Design review of the part shown in the three views and the two pictorial views. Dimensions are in mm from the part's minimum x, y and z. Round coordinates to 2 decimals unless told otherwise and drop trailing zeros. Order: outer loops, then holes, each group sorted by start corner. A loop starts at its lowest first (then second) coordinate and runs counter-clockwise, first axis right, second up.
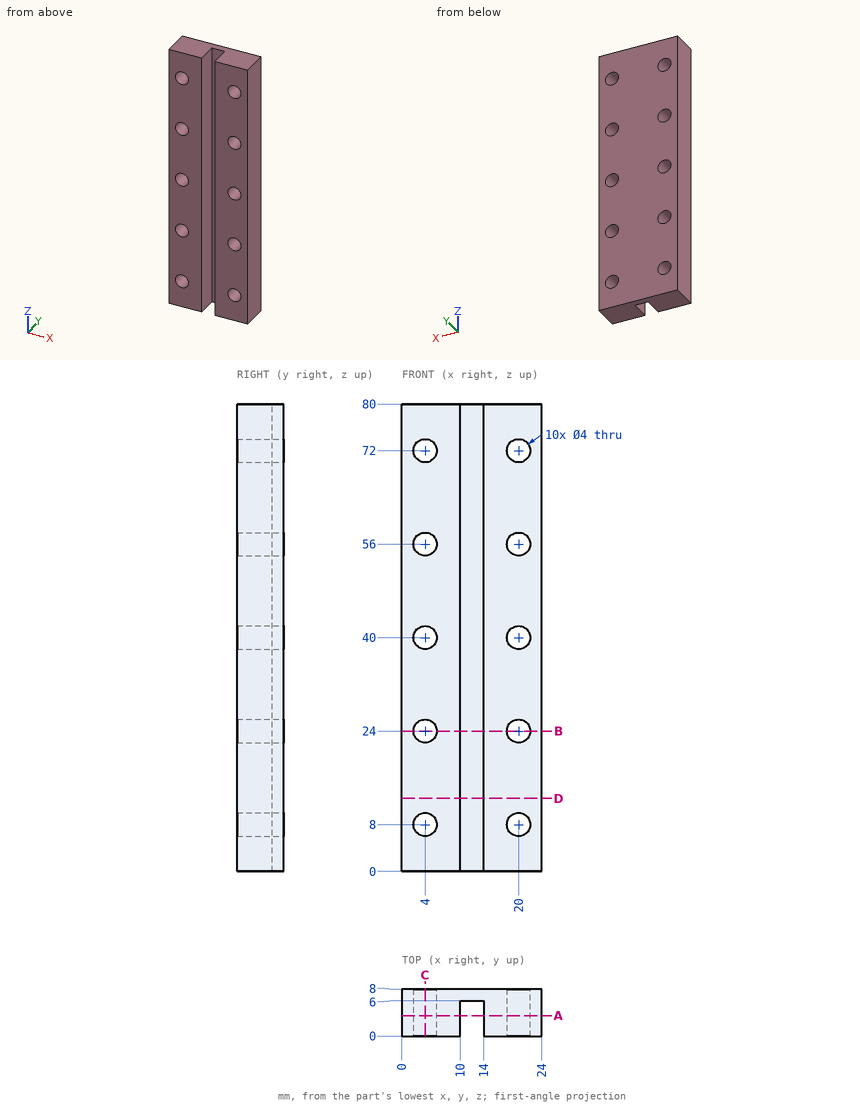
(1) Clearance check with flat-ended pins moving along their axes: P1, Ø3.5, axis at x = 4, z = 40, coming from the +Y side; P2, Ø1.2, axis at x = 12, z = 25.5, coming from the -Y side. State where each tip first meets the part, or that it passes through.
(2) Add section B-B on z = 24. Give the boundary of the cut face in (x, y).
(3) Add section D-D on z = 12.5. Give the boundary of the cut face in (x, y), plus the area to 3 significant figures.
(4) Add section C-C on x = 4. Give the boundary of the cut face in (y, z).
(5) Add section A-A on y = 3.5. Count the separate pieces of the cut face and the enclosed holes in it, plus the area to 3 significant figures.
(6) Wall thickness on L1, parallel to Z at x = 4, y = 2; L2, parallel to X at y = 0.5, z = 77.5; L3, parallel to X at y = 3.5, z = 8.5: over which ranges is each line inside the solid? List them lowest first.
Here are the results:
1. P1: passes through
1. P2: stops at y = 6
2. outline: (0, 0) - (2, 0) - (2, 8) - (0, 8) - close; (6, 0) - (10, 0) - (10, 6) - (14, 6) - (14, 0) - (18, 0) - (18, 8) - (6, 8) - close; (22, 0) - (24, 0) - (24, 8) - (22, 8) - close
3. outline: (0, 0) - (10, 0) - (10, 6) - (14, 6) - (14, 0) - (24, 0) - (24, 8) - (0, 8) - close
3. area: 168 mm2
4. outline: (0, 0) - (8, 0) - (8, 6) - (0, 6) - close; (0, 10) - (8, 10) - (8, 22) - (0, 22) - close; (0, 26) - (8, 26) - (8, 38) - (0, 38) - close; (0, 42) - (8, 42) - (8, 54) - (0, 54) - close; (0, 58) - (8, 58) - (8, 70) - (0, 70) - close; (0, 74) - (8, 74) - (8, 80) - (0, 80) - close
5. separate pieces: 2
5. enclosed holes: 10
5. area: 1,470 mm2
6. L1: z = 0 to 6, 10 to 22, 26 to 38, 42 to 54, 58 to 70, 74 to 80
6. L2: x = 0 to 10, 14 to 24
6. L3: x = 0 to 2.06, 5.94 to 10, 14 to 18.06, 21.94 to 24
